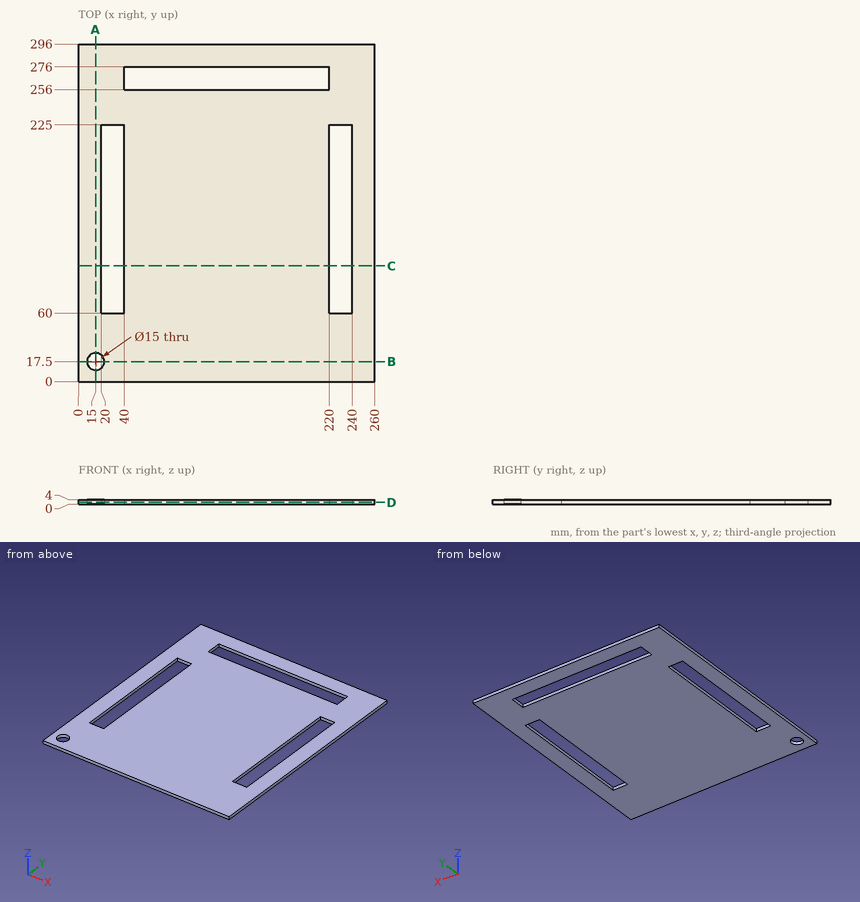
Study the drawing (mm; zero at the part's minimum x, y, z) and answer. Coordinates: 2 decimals unless noted, no trailing zeros. Order: outer loops, then holes, each group sorted by start corner. A loop starts at its lowest first (then second) coordinate and runs counter-clockwise, first axis right, second up. Notation, with made-up numbers: (-5.5, 17.5) -> (40.5, 17.5) arc R23 ccw to (40.5, 37.5) -> close; hole circle Ø9 at (74.5, 29). An arc over 180 degrees is marked (long way). Answer in a Markdown table with one row per item. Add a question column.
Item 1: Find section B-B (y = 17.5). Write down the section's boundary in (x, z).
Item 2: Find section A-A (x = 15). Write down the section's boundary in (y, z), then the cut area to 3 significant figures.
Item 3: Find section D-D (z = 1.55). Write down the section's boundary in (x, y), then the cut area to 3 significant figures.
Item 4: Find section C-C (y = 101.5). Write down the section's boundary in (x, z), then the cut area to 3 significant figures.
Item 5: This flat-tipped pin is pushed along its axis until it touches: P1, Ø2, axis at x = 226, z = 1, coming from the -Y side. Where does it stop, or does it pass through?
Item 6: Find the intervals of material crossed by L1, parallel to X at y = 159, z = 2; L2, parallel to Y at x = 222.5, z = 1.7; L3, parallel to Y at x = 15, z = 2.8, in increasing order. Write a range as from..to.
Result set:
| question | item | result |
|---|---|---|
| 1 | outline | (0, 0) -> (7.5, 0) -> (7.5, 4) -> (0, 4) -> close; (22.5, 0) -> (260, 0) -> (260, 4) -> (22.5, 4) -> close |
| 2 | outline | (0, 0) -> (10, 0) -> (10, 4) -> (0, 4) -> close; (25, 0) -> (296, 0) -> (296, 4) -> (25, 4) -> close |
| 2 | area | 1,120 mm² |
| 3 | outline | (0, 0) -> (260, 0) -> (260, 296) -> (0, 296) -> close; hole circle Ø15 at (15, 17.5); hole (20, 60) -> (40, 60) -> (40, 225) -> (20, 225) -> close; hole (40, 256) -> (220, 256) -> (220, 276) -> (40, 276) -> close; hole (220, 60) -> (240, 60) -> (240, 225) -> (220, 225) -> close |
| 3 | area | 66,600 mm² |
| 4 | outline | (0, 0) -> (20, 0) -> (20, 4) -> (0, 4) -> close; (40, 0) -> (220, 0) -> (220, 4) -> (40, 4) -> close; (240, 0) -> (260, 0) -> (260, 4) -> (240, 4) -> close |
| 4 | area | 880 mm² |
| 5 | P1 | stops at y = 0 |
| 6 | L1 | x = 0..20, 40..220, 240..260 |
| 6 | L2 | y = 0..60, 225..296 |
| 6 | L3 | y = 0..10, 25..296 |
